Read the model definition and answer for the solid it produces. Units are mm, in the model's axes. Give positions to 0.01 mm unless a question says otherwise; leave off trailing zeros. Order: outer loops, then holes, each group sorted by start corner. A loop starts at its lowest first (then second) coordinate and runs counter-clockwise, first axis right, second up. Notation, with made-up numbers: (-17.5, -21.75) - (8.5, -21.75) arc R28 ccw to (8.5, 11.25) - close; hole circle Ø3 at (60.25, -39.75). An arc over 180 degrees is marked (long way). Use a Markdown table: item, result. Add a question column.
1. A flat-ended cylindrical pin translates along its axis: P1, Ø1, axis at x = 10, z = -2, coming from the +Y side. Find the tip coordinate at first contact, or state that the pin passes through.
2. Consider L1, parallel to Z at x = 0, y = 0.3; L2, parallel to X at y = 0.2, z = 0; L3, parallel to X at y = 0.2, z = 0.75. Determine where each line is inside the solid, lowest interval first.
3. A cutting plane is placed at D-D on z = 2.5. Determine the outline of the cut face in (x, y).
4. A cutting plane is placed at B-B on z = -0.75. Determine the outline of the cut face in (x, y), and give its area (3 significant figures).
5. A cutting plane is placed at C-C on x = 6.75. Determine the outline of the cut face in (y, z), and give its area (3 significant figures).
6. A cutting plane is placed at A-A on x = 0. Determine the outline of the cut face in (y, z).
7. For a pull along Z with two mould halves and no side action, classify faces 1 (the flat face through (1.3, 0.5, 0)), 2 (the cylindrical face through (0.085, 0.246, -4.007)), 3 (the cylindrical face through (-0.217, 0.254, 0.976)), 4 (the cylindrical face through (-0.085, 0.246, 4.007)) as released by +Z, released by -Z, zero draft, split by the parting line, or undercut.
```python
from build123d import *

# Parameters (mm, degrees)
BOSS_EXTRUDE2_DEPTH = 0.5
SKETCH3_R           = 1
CUT_EXTRUDE2_DEPTH  = 1.5000001


with BuildPart() as part:
    # Sketch1 → Boss-Extrude2 (new body)
    with BuildSketch(Plane(origin=(0, 0, 0), x_dir=(1, 0, 0), z_dir=(0, 1, 0))):
        with BuildLine():
            Line((15.859342687, 0.25), (4, 0.25))
            ThreePointArc((4, 0.25), (0, 4.007804885), (-4, 0.25))
            Line((-4, 0.25), (-8.33886799, 0.428130321))
            add(Edge.make_bspline(
                [(-8.33886799, 0.428130321), (-9.480171403, 0), (-8.33886799, -0.428130321)],
                knots=[0, 0, 0, 1, 1, 1], degree=2))
            Line((-8.33886799, -0.428130321), (-4, -0.25))
            ThreePointArc((-4, -0.25), (0, -4.007804885), (4, -0.25))
            Line((4, -0.25), (15.859342687, -0.25))
            Line((15.859342687, -0.25), (15.859342687, 0.25))
        make_face()
    extrude(amount=BOSS_EXTRUDE2_DEPTH)

    # Sketch3 → Cut-Extrude2 (cut, through all)
    with BuildSketch(Plane(origin=(0, 0.5, 0), x_dir=(1, 0, 0), z_dir=(0, 1, 0))):
        Circle(SKETCH3_R)
    extrude(amount=-CUT_EXTRUDE2_DEPTH, mode=Mode.SUBTRACT)


solid = part.part
```
Output values:
| question | item | result |
|---|---|---|
| 1 | P1 | through |
| 2 | L1 | -4.01 to -1, 1 to 4.01 |
| 2 | L2 | -8.91 to -1, 1 to 15.86 |
| 2 | L3 | -3.94 to -0.66, 0.66 to 3.94 |
| 3 | outline | (-3.13, 0) - (3.13, 0) - (3.13, 0.5) - (-3.13, 0.5) - close |
| 4 | outline | (-3.94, 0) - (-0.66, 0) - (-0.66, 0.5) - (-3.94, 0.5) - close; (0.66, 0) - (3.94, 0) - (3.94, 0.5) - (0.66, 0.5) - close |
| 4 | area | 3.28 mm² |
| 5 | outline | (0, -0.25) - (0.5, -0.25) - (0.5, 0.25) - (0, 0.25) - close |
| 5 | area | 0.250 mm² |
| 6 | outline | (0, -4.01) - (0.5, -4.01) - (0.5, -1) - (0, -1) - close; (0, 1) - (0.5, 1) - (0.5, 4.01) - (0, 4.01) - close |
| 7 | face 1 | zero draft |
| 7 | face 2 | released by -Z |
| 7 | face 3 | undercut |
| 7 | face 4 | released by +Z |
